```python
from build123d import *

# Parameters (mm, degrees)
F0_W          = 124.7
F0_H          = 107
F0_W_2        = 122
F0_H_2        = 102
F0_W_3        = 1.3
F1_DEPTH      = 2
F2_DEPTH      = 20
F3_DEPTH      = 1.5
F3_DEPTH_BACK = 2


with BuildPart() as f1:
    # F0 (on Front) → F1 (new body)
    with BuildSketch(Plane.XZ):
        Polygon((-78.3, -61.5), (66.5, -61.5), (66.5, -60.5), (61.7, -60.5), (61.7, -55.5), (-65, -55.5), (-65, 55.5), (61.7, 55.5), (61.7, 60.5), (66.5, 60.5), (66.5, 61.5), (-78.3, 61.5), align=None)
        Polygon((61.7, -53.5), (61.7, -55.5), (65, -55.5), (65, 55.5), (61.7, 55.5), (61.7, 53.5), (63, 53.5), (63, -53.5), align=None)
        Polygon((-65, -55.5), (61.7, -55.5), (61.7, -53.5), (-63, -53.5), (-63, 53.5), (61.7, 53.5), (61.7, 55.5), (-65, 55.5), align=None)
        with Locations((-0.65, 0)):
            Rectangle(F0_W, F0_H)
        with Locations((-0.3, 0)):
            Rectangle(F0_W_2, F0_H_2, mode=Mode.SUBTRACT)
        Polygon((61.7, -60.5), (66.5, -60.5), (66.5, 60.5), (61.7, 60.5), (61.7, 55.5), (65, 55.5), (65, -55.5), (61.7, -55.5), align=None)
        with Locations((62.35, 0)):
            Rectangle(F0_W_3, F0_H)
    extrude(amount=-F1_DEPTH)

    # F0 (on Front) → F2 (join)
    with BuildSketch(Plane.XZ):
        Polygon((61.7, -53.5), (61.7, -55.5), (65, -55.5), (65, 55.5), (61.7, 55.5), (61.7, 53.5), (63, 53.5), (63, -53.5), align=None)
        Polygon((-65, -55.5), (61.7, -55.5), (61.7, -53.5), (-63, -53.5), (-63, 53.5), (61.7, 53.5), (61.7, 55.5), (-65, 55.5), align=None)
    extrude(amount=-F2_DEPTH)

    # F0 (on Front) → F3 (cut, two sides)
    with BuildSketch(Plane.XZ) as f3_sk:
        Polygon((61.7, -60.5), (66.5, -60.5), (66.5, 60.5), (61.7, 60.5), (61.7, 55.5), (65, 55.5), (65, -55.5), (61.7, -55.5), align=None)
        with Locations((62.35, 0)):
            Rectangle(F0_W_3, F0_H)
        Polygon((61.7, -53.5), (61.7, -55.5), (65, -55.5), (65, 55.5), (61.7, 55.5), (61.7, 53.5), (63, 53.5), (63, -53.5), align=None)
    extrude(amount=-F3_DEPTH, mode=Mode.SUBTRACT)
    extrude(f3_sk.sketch, amount=F3_DEPTH_BACK, mode=Mode.SUBTRACT)


solid = f1.part
```
Verification items for the finished model (mm, model axes). A direction names the side the tool comes from. Coordinates: 2 decimals unless noted, no trailing zeros. Loops run counter-clockwise (first coordinate to the right, second up) from the corner with the lowest first, then second, coordinate; pieces in that order, holes last. Notation, with made-up numbers: (-24, 56) - (11, 56) arc R24 cw to (11, 72) - close; hole circle Ø1 at (-4.5, -18). An arc over 180 degrees is marked (long way). Return JSON: item names as keys, results as strings.
1. Thickness scan on L1, parallel to X at y = 14, z = 39; L2, parallel to Z at x = 41.5, y = 1.75; L3, parallel to Z at x = -42, y = 4.25. Record the ranges inside material, lowest first.
Established:
{"L1": "x = -65 to -63, 63 to 65", "L2": "z = -61.5 to -51, 51 to 61.5", "L3": "z = -55.5 to -53.5, 53.5 to 55.5"}
2. Mould release check, pull along Z, two halves, no side actions. Record for faces 6 (the flat face through (1, 11, 55.5)), 7 (the flat face through (-1, 11, -55.5)), 8 (the flat face through (64, 1.5, 1)): +Z half, -Z half, draft (parallel to the pull), parting line (faces both ways), or undercut.
Established:
{"face 6": "+Z half", "face 7": "-Z half", "face 8": "undercut"}
3. Section check A-A, the plane z = 34. Record the boundary of the cut face in (x, y), then the cut area to 3 significant figures.
Established:
{"outline": "(-78.3, 0) - (-61.3, 0) - (-61.3, 2) - (-63, 2) - (-63, 20) - (-65, 20) - (-65, 2) - (-78.3, 2) - close; (60.7, 0) - (61.7, 0) - (61.7, 1.5) - (66.5, 1.5) - (66.5, 2) - (65, 2) - (65, 20) - (63, 20) - (63, 2) - (60.7, 2) - close", "area": "110 mm2"}
4. Section check B-B, the plane y = 6.5. Record the boundary of the cut face in (x, z).
Established:
{"outline": "(-65, -55.5) - (65, -55.5) - (65, 55.5) - (-65, 55.5) - close; hole (-63, -53.5) - (63, -53.5) - (63, 53.5) - (-63, 53.5) - close"}
5. Section check C-C, the plane x = 16. Record the boundary of the cut face in (y, z), then the cut area to 3 significant figures.
Established:
{"outline": "(0, -61.5) - (2, -61.5) - (2, -55.5) - (20, -55.5) - (20, -53.5) - (2, -53.5) - (2, -51) - (0, -51) - close; (0, 51) - (2, 51) - (2, 53.5) - (20, 53.5) - (20, 55.5) - (2, 55.5) - (2, 61.5) - (0, 61.5) - close", "area": "114 mm2"}
6. Go/stop test with flat-tipped pins: pin 1 (1 mm diameter, centred on x = 39.5, y = 10, fed in from -Z); pin 2 (1.6 mm diameter, centred on y = 0.5, z = 20.5, fed in from +X); pin 3 (4 mm diameter, centred on x = 64, z = 6, fed in from -Y). Record where each tip stops, or that it passes through.
Established:
{"pin 1": "stops at z = -55.5", "pin 2": "stops at x = 61.7", "pin 3": "stops at y = 1.5"}
7. Tool access check on faces 1 (the flat face through (0, 20, 54)), 2 (the flat face through (-65, 11, 1)), 3 (the flat face through (0, 2, 52)), 4 (the flat face through (-65, 0, 0)), 5 (the flat face through (65, 11, -1)). Record the directions out of +Z, -Z, +X, -X, +Y, -Y that give a thin tool (end or side, any length) a straight path to the whole face; none if there is none.
Established:
{"face 1": "+Z, -Z, +X, -X, +Y", "face 2": "+Z, -Z, -X, +Y", "face 3": "+Y", "face 4": "+Z, -Z, +X, -X, -Y", "face 5": "+Z, -Z, +X, +Y"}
